```python
from build123d import *

# Parameters (mm, degrees)
SKETCH1_W                = 49.9
SKETCH1_H                = 49.9
BOSS_EXTRUDE1_DEPTH      = 6
BOSS_EXTRUDE2_DEPTH      = 5.9
SKETCH3_R                = 1.5
BOSS_EXTRUDE3_DEPTH      = 13
BOSS_EXTRUDE3_DEPTH_BACK = 14.9
SKETCH4_R                = 2.5
BOSS_EXTRUDE4_DEPTH      = 5
SKETCH5_R                = 1.5
BOSS_EXTRUDE5_DEPTH      = 3
SKETCH6_R                = 2.75
BOSS_EXTRUDE6_DEPTH      = 0.5
SKETCH7_R                = 2.75
BOSS_EXTRUDE7_DEPTH      = 2.5
SKETCH8_W                = 33
SKETCH8_H                = 33
SKETCH8_R                = 8.675
BOSS_EXTRUDE8_DEPTH      = 1
SKETCH9_W                = 33
SKETCH9_H                = 33
SKETCH9_R                = 10.15
BOSS_EXTRUDE9_DEPTH      = 7
SKETCH10_R               = 10
BOSS_EXTRUDE10_DEPTH     = 2
SKETCH11_R               = 10.15
SKETCH11_R_2             = 6
BOSS_EXTRUDE11_DEPTH     = 3
SKETCH12_R               = 2
CUT_EXTRUDE1_DEPTH       = 13
SKETCH13_R               = 4
CUT_EXTRUDE2_DEPTH       = 4
SKETCH14_R               = 3.5
BOSS_EXTRUDE12_DEPTH     = 1
SKETCH15_R               = 3.5
BOSS_EXTRUDE13_DEPTH     = 3
BOSS_EXTRUDE14_DEPTH     = 13
SKETCH17_R               = 8
CUT_EXTRUDE3_DEPTH       = 3
CHAMFER1_SIZE            = 1
SKETCH18_R               = 2.75
BOSS_EXTRUDE15_DEPTH     = 0.5
SKETCH19_R               = 2.75
BOSS_EXTRUDE16_DEPTH     = 2.5


with BuildPart() as part:
    # Sketch1 → Boss-Extrude1 (new body)
    with BuildSketch(Plane(origin=(0, -32.5, 0), x_dir=(1, 0, 0), z_dir=(0, 1, 0))):
        with Locations((-9.95, -9.95)):
            Rectangle(SKETCH1_W, SKETCH1_H)
        with BuildLine():
            Line((1.05, 8.3), (10.05, 8.3))
            ThreePointArc((10.05, 8.3), (12.55, 5.8), (10.05, 3.3))
            Line((10.05, 3.3), (1.05, 3.3))
            ThreePointArc((1.05, 3.3), (-1.45, 5.8), (1.05, 8.3))
        make_face(mode=Mode.SUBTRACT)
        with BuildLine():
            Line((-20.95, 8.3), (-29.95, 8.3))
            ThreePointArc((-29.95, 8.3), (-32.45, 5.8), (-29.95, 3.3))
            Line((-29.95, 3.3), (-20.95, 3.3))
            ThreePointArc((-20.95, 3.3), (-18.45, 5.8), (-20.95, 8.3))
        make_face(mode=Mode.SUBTRACT)
        with BuildLine():
            Line((-20.95, -28.2), (-29.95, -28.2))
            ThreePointArc((-29.95, -28.2), (-32.45, -25.7), (-29.95, -23.2))
            Line((-29.95, -23.2), (-20.95, -23.2))
            ThreePointArc((-20.95, -23.2), (-18.45, -25.7), (-20.95, -28.2))
        make_face(mode=Mode.SUBTRACT)
        with BuildLine():
            Line((1.05, -28.2), (10.05, -28.2))
            ThreePointArc((10.05, -28.2), (12.55, -25.7), (10.05, -23.2))
            Line((10.05, -23.2), (1.05, -23.2))
            ThreePointArc((1.05, -23.2), (-1.45, -25.7), (1.05, -28.2))
        make_face(mode=Mode.SUBTRACT)
    extrude(amount=-BOSS_EXTRUDE1_DEPTH)

    # Sketch2 → Boss-Extrude2 (add)
    with BuildSketch(Plane(origin=(-6.363961031, 0, 6.363961031), x_dir=(0, -1, 0), z_dir=(0.707106781, 0, -0.707106781))):
        with BuildLine():
            Line((-5.545268253, -9.5), (-17.25, -9.5))
            Line((-17.25, -9.5), (-17.25, -16.5))
            Line((-17.25, -16.5), (32.5, -16.5))
            Line((32.5, -16.5), (32.5, 16.5))
            Line((32.5, 16.5), (8.9, 16.5))
            Line((8.9, 16.5), (8.9, 6.464518544))
            ThreePointArc((8.9, 6.464518544), (8.156593612, -7.380378083), (-5.545268253, -9.5))
        make_face()
    extrude(amount=-BOSS_EXTRUDE2_DEPTH)

    # Sketch3 → Boss-Extrude3 (add, two sides)
    with BuildSketch(Plane(origin=(-10.53589104, 0, 10.53589104), x_dir=(0.707106781, 0, 0.707106781), z_dir=(-0.707106781, 0, 0.707106781))) as boss_extrude3_sk:
        with Locations((13.25, 13.25)):
            Circle(SKETCH3_R)
        with Locations((13.25, -13.25)):
            Circle(SKETCH3_R)
        with Locations((-13.25, -13.25)):
            Circle(SKETCH3_R)
    extrude(amount=BOSS_EXTRUDE3_DEPTH)
    extrude(boss_extrude3_sk.sketch, amount=-BOSS_EXTRUDE3_DEPTH_BACK)

    # Sketch4 → Boss-Extrude4 (add)
    with BuildSketch(Plane(origin=(-19.728279195, 0, 19.728279195), x_dir=(0.707106781, 0, 0.707106781), z_dir=(-0.707106781, 0, 0.707106781))):
        with Locations((13.25, 13.25)):
            Circle(SKETCH4_R)
        with Locations((13.25, -13.25)):
            Circle(SKETCH4_R)
        with Locations((-13.25, -13.25)):
            Circle(SKETCH4_R)
    extrude(amount=-BOSS_EXTRUDE4_DEPTH)

    # Sketch5 → Boss-Extrude5 (add)
    with BuildSketch(Plane(origin=(-10.53589104, 0, 10.53589104), x_dir=(0.707106781, 0, 0.707106781), z_dir=(-0.707106781, 0, 0.707106781))):
        with Locations((-7.25, -13.25)):
            Circle(SKETCH5_R)
        with Locations((13.25, 7.25)):
            Circle(SKETCH5_R)
    extrude(amount=BOSS_EXTRUDE5_DEPTH)

    # Sketch6 → Boss-Extrude6 (add)
    with BuildSketch(Plane(origin=(-12.657211383, 0, 12.657211383), x_dir=(0.707106781, 0, 0.707106781), z_dir=(-0.707106781, 0, 0.707106781))):
        with Locations((13.25, 7.25)):
            Circle(SKETCH6_R)
        with Locations((-7.25, -13.25)):
            Circle(SKETCH6_R)
    extrude(amount=BOSS_EXTRUDE6_DEPTH)

    # Sketch7 → Boss-Extrude7 (add)
    with BuildSketch(Plane(origin=(-13.010764774, 0, 13.010764774), x_dir=(0.707106781, 0, 0.707106781), z_dir=(-0.707106781, 0, 0.707106781))):
        with Locations((-7.25, -13.25)):
            Circle(SKETCH7_R)
        Polygon((-6.221372178, -12.237449687), (-7.612580383, -11.852907018), (-8.641208205, -12.865457332), (-8.278627822, -14.262550313), (-6.887419617, -14.647092982), (-5.858791795, -13.634542668), align=None, mode=Mode.SUBTRACT)
        with Locations((13.25, 7.25)):
            Circle(SKETCH7_R)
        Polygon((13.787086733, 5.910271978), (14.678781868, 7.045266744), (14.141695135, 8.384994766), (12.712913267, 8.589728022), (11.821218132, 7.454733256), (12.358304865, 6.115005234), align=None, mode=Mode.SUBTRACT)
    extrude(amount=BOSS_EXTRUDE7_DEPTH)

    # Sketch8 → Boss-Extrude8 (add)
    with BuildSketch(Plane(origin=(0, 0, 0), x_dir=(0, -1, 0), z_dir=(0.707106781, 0, -0.707106781))):
        Rectangle(SKETCH8_W, SKETCH8_H)
        Circle(SKETCH8_R, mode=Mode.SUBTRACT)
    extrude(amount=BOSS_EXTRUDE8_DEPTH)

    # Sketch9 → Boss-Extrude9 (add)
    with BuildSketch(Plane(origin=(0, 0, 0), x_dir=(0.707106781, 0, 0.707106781), z_dir=(-0.707106781, 0, 0.707106781))):
        Rectangle(SKETCH9_W, SKETCH9_H)
        Circle(SKETCH9_R, mode=Mode.SUBTRACT)
    extrude(amount=BOSS_EXTRUDE9_DEPTH)

    # Sketch10 → Boss-Extrude10 (add)
    with BuildSketch(Plane(origin=(0, 0, 0), x_dir=(0.707106781, 0, 0.707106781), z_dir=(-0.707106781, 0, 0.707106781))):
        Circle(SKETCH10_R)
    extrude(amount=BOSS_EXTRUDE10_DEPTH)

    # Sketch11 → Boss-Extrude11 (add)
    with BuildSketch(Plane(origin=(-1.414213562, 0, 1.414213562), x_dir=(0.707106781, 0, 0.707106781), z_dir=(-0.707106781, 0, 0.707106781))):
        Circle(SKETCH11_R)
        Circle(SKETCH11_R_2, mode=Mode.SUBTRACT)
    extrude(amount=BOSS_EXTRUDE11_DEPTH)

    # Sketch12 → Cut-Extrude1 (cut)
    with BuildSketch(Plane.XZ.offset(38.5)):
        with Locations((-15.344217152, 1.555634919)):
            Circle(SKETCH12_R)
        with Locations((-1.555634919, 15.344217152)):
            Circle(SKETCH12_R)
    extrude(amount=-CUT_EXTRUDE1_DEPTH, mode=Mode.SUBTRACT)

    # Sketch13 → Cut-Extrude2 (cut)
    with BuildSketch(Plane.XZ.offset(38.5)):
        with Locations((-15.344217152, 1.555634919)):
            Circle(SKETCH13_R)
        with Locations((-1.555634919, 15.344217152)):
            Circle(SKETCH13_R)
    extrude(amount=-CUT_EXTRUDE2_DEPTH, mode=Mode.SUBTRACT)

    # Sketch14 → Boss-Extrude12 (add)
    with BuildSketch(Plane.XZ.offset(34.5)):
        with Locations((-15.344217152, 1.555634919)):
            Circle(SKETCH14_R)
        with Locations((-1.555634919, 15.344217152)):
            Circle(SKETCH14_R)
    extrude(amount=BOSS_EXTRUDE12_DEPTH)

    # Sketch15 → Boss-Extrude13 (add)
    with BuildSketch(Plane.XZ.offset(35.5)):
        with Locations((-1.555634919, 15.344217152)):
            Circle(SKETCH15_R)
        Polygon((-2.665434879, 16.674008131), (-3.262167668, 15.047997683), (-2.152367708, 13.718206703), (-0.445834958, 14.014426173), (0.150897831, 15.640436621), (-0.958902129, 16.9702276), align=None, mode=Mode.SUBTRACT)
        with Locations((-15.344217152, 1.555634919)):
            Circle(SKETCH15_R)
        Polygon((-14.297928697, 2.935953893), (-16.016464221, 3.151906787), (-17.062752676, 1.771587813), (-16.390505606, 0.175315945), (-14.671970082, -0.04063695), (-13.625681628, 1.339682024), align=None, mode=Mode.SUBTRACT)
    extrude(amount=BOSS_EXTRUDE13_DEPTH)

    # Sketch16 → Boss-Extrude14 (add, symmetric)
    with BuildSketch(Plane(origin=(0, 0, 0), x_dir=(1, 0, 0), z_dir=(0, 1, 0))):
        Polygon((-10.960155108, 12.374368671), (-16.263455967, 7.071067812), (-18.384776311, 9.192388155), (-12.202795796, 15.374368671), (10.289844892, 15.374368671), (10.289844892, 12.374368671), align=None)
    extrude(amount=BOSS_EXTRUDE14_DEPTH, both=True)

    # Sketch17 → Cut-Extrude3 (cut)
    with BuildSketch(Plane(origin=(0, 0, -15.374368671), x_dir=(-1, 0, 0), z_dir=(0, 0, -1))):
        Circle(SKETCH17_R)
    extrude(amount=-CUT_EXTRUDE3_DEPTH, mode=Mode.SUBTRACT)

    # Chamfer1
    chamfer1_edges = [part.edges().sort_by_distance(p)[0] for p in [
        (8, 0, -12.374368671),
        (8, 0, -15.374368671),
    ]]
    chamfer(chamfer1_edges, length=CHAMFER1_SIZE)

    # Sketch18 → Boss-Extrude15 (add)
    with BuildSketch(Plane(origin=(-13.788582233, 0, -13.788582233), x_dir=(-0.707106781, 0, 0.707106781), z_dir=(-0.707106781, 0, -0.707106781))):
        with Locations((3, 10)):
            Circle(SKETCH18_R)
        with Locations((3, -10)):
            Circle(SKETCH18_R)
    extrude(amount=BOSS_EXTRUDE15_DEPTH)

    # Sketch19 → Boss-Extrude16 (add)
    with BuildSketch(Plane(origin=(-14.142135624, 0, -14.142135624), x_dir=(-0.707106781, 0, 0.707106781), z_dir=(-0.707106781, 0, -0.707106781))):
        with Locations((3, -10)):
            Circle(SKETCH19_R)
        Polygon((3.666920263, -11.280058865), (4.442023626, -10.062459543), (3.775103364, -8.782400678), (2.333079737, -8.719941135), (1.557976374, -9.937540457), (2.224896636, -11.217599322), align=None, mode=Mode.SUBTRACT)
        with Locations((3, 10)):
            Circle(SKETCH19_R)
        Polygon((1.848210491, 9.130106754), (3.177454895, 8.567574402), (4.329244404, 9.437467649), (4.151789509, 10.869893246), (2.822545105, 11.432425598), (1.670755596, 10.562532351), align=None, mode=Mode.SUBTRACT)
    extrude(amount=BOSS_EXTRUDE16_DEPTH)


solid = part.part
```
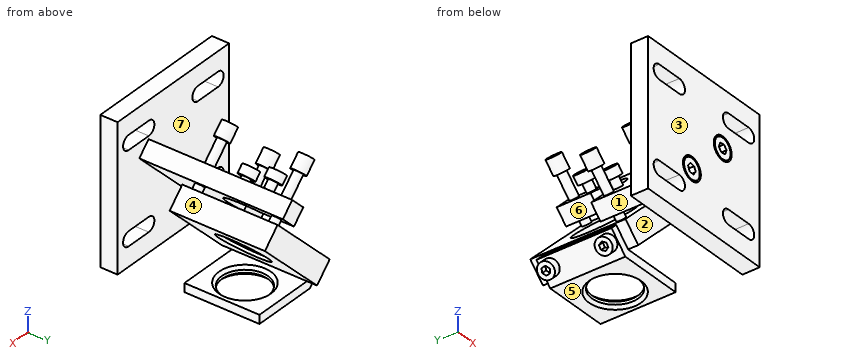
Verification items for the finished model (mm, model axes). Face numbers are marked on the shaded views. A direction names the side the tool comes from. Round coordinates to 2 decimals unless told otherwise and drop trailing zeros. Write each loop counter-clockwise with the first axis right and the second up, starting at its lowest first coordinate (ties: lowest second). Pieces come first, ordered by that corner, then holes. Notation, with made-up numbers: (79.5, 49.25) -> (98.5, 49.25) arc R21 cw to (98.5, 71.25) -> close; hole circle Ø6 at (11, 50). An arc over 180 degrees is marked (long way). Write each question's results on one line, items separated by ' | '. Start each with the question number.
1. Depth check by flat-ended pin: P1, Ø3, axis at x = 6.5, y = 9.5, coming from the -Z side; P2, Ø6, axis at x = -7.5, z = 24.5, coming from the +Y side; P3, Ø3, axis at x = -16.5, z = 1, coming from the +Y side. Enter the tip coordinate at first touch or a pass-through.
2. Draft check along Y on the marked faces 1, 2 and 3. Enter one of: +Y half, -Y half, draft (parallel to the pull), parting line (faces both ways), or undercut.
3. Cross-section at A-A (y = -33.5). Enter the section's corners in (x, z), then the cut area to 3 significant figures.
4. Cross-section at B-B (y = -21.5). Enter the section's corners in (x, z).
5. Material ranges on probe 1 along Y at (x, z) = (4, 11); probe 2 along Y at (x, z) = (-17, -10.5); probe 3 along Z at (x, y) = (-6, -6), recorded low to high. Write a range as from..to.
6. Set-up check for the marked faces 4, 5, 6 and 7: record each of +Z, -Z, +X, -X, +Y, -Y from which the full face is reachable in a straight line by a thin tool's end or side.
7. Cross-section at C-C (y = 0). Count the separate pieces of the cut face and the enclosed holes in it, then the cut area to 3 significant figures.
Solutions:
1) P1: stops at z = -15.37 | P2: stops at y = 15.75 | P3: stops at y = -8.9
2) face 1: draft | face 2: undercut | face 3: -Y half
3) outline: (-34.9, -15) -> (15, -15) -> (15, 34.9) -> (-34.9, 34.9) -> close; hole (-29.95, -8.3) -> (-20.95, -8.3) arc R2.5 ccw to (-20.95, -3.3) -> (-29.95, -3.3) arc R2.5 ccw to start; hole (-29.95, 23.2) -> (-20.95, 23.2) arc R2.5 ccw to (-20.95, 28.2) -> (-29.95, 28.2) arc R2.5 ccw to start; hole circle Ø4 at (-15.34, 1.56); hole circle Ø4 at (-1.56, 15.34); hole (1.05, -8.3) -> (10.05, -8.3) arc R2.5 ccw to (10.05, -3.3) -> (1.05, -3.3) arc R2.5 ccw to start; hole (1.05, 23.2) -> (10.05, 23.2) arc R2.5 ccw to (10.05, 28.2) -> (1.05, 28.2) arc R2.5 ccw to start | area: 2,210 mm2
4) outline: (-22.2, -1.13) -> (-18.03, -5.3) -> (5.3, 18.03) -> (1.13, 22.2) -> close
5) probe 1: y = -38.5..-32.5, -16.5..16.5 | probe 2: y = -38.5..-32.5, -13..13 | probe 3: z = -14.86..-12.89, -7.41..-5.58, -5.31..1.07
6) face 4: +Z, +X, +Y | face 5: -Z, +X, +Y, -Y | face 6: -X, +Y | face 7: none
7) separate pieces: 3 | enclosed holes: 2 | area: 242 mm2
